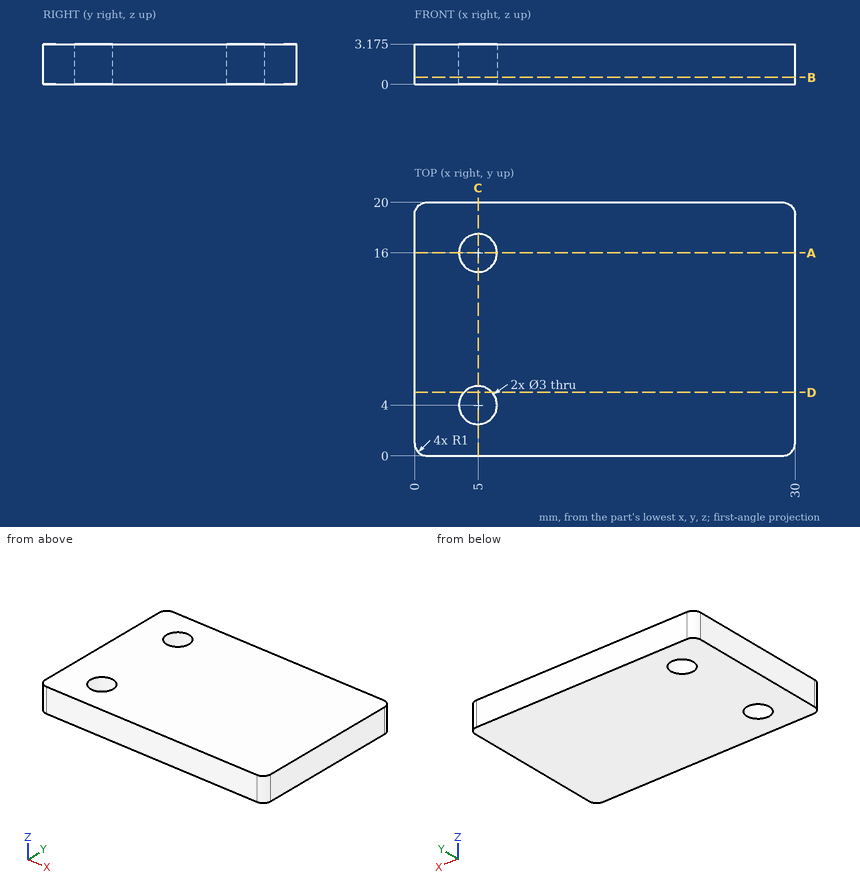
Study the drawing (mm; zero at the part's minimum x, y, z) and answer. Give positions to 0.01 mm unless a question says otherwise; leave off trailing zeros. Write each loop counter-clockwise with the first axis right and the second up, starting at its lowest first coordinate (ties: lowest second). Pieces come first, ordered by that corner, then holes. Notation, with made-up numbers: (-13, -1.5) - (7, -1.5) arc R24 ccw to (7, 10.5) - close; hole circle Ø11 at (69, 34.5). An arc over 180 degrees is marked (long way). One line per question, with ' | ' between items. Start each with the question number.
1. Section D-D, the plane y = 5 is taken. Determine the outline of the cut face in (x, z) (3 decimals), then the cut area to 3 significant figures.
2. Section B-B, the plane z = 0.55 is taken. Determine the outline of the cut face in (x, y), then the cut area to 3 significant figures.
3. Straight lines are drawn through the part: line 1 (Y direction, x = 5, z = 1.7); line 2 (X direction, y = 2.75, z = 3.05); line 3 (X direction, y = 16.75, z = 1.6). For each, find the intervals that lie inside material, in ascending order.
4. Section C-C, the plane x = 5 is taken. Determine the outline of the cut face in (y, z) (3 decimals).
5. Section A-A, the plane y = 16 is taken. Determine the outline of the cut face in (x, z) (3 decimals), then the cut area to 3 significant figures.
Result:
1) outline: (0, 0) - (3.882, 0) - (3.882, 3.175) - (0, 3.175) - close; (6.118, 0) - (30, 0) - (30, 3.175) - (6.118, 3.175) - close | area: 88.2 mm2
2) outline: (0, 1) arc R1 ccw to (1, 0) - (29, 0) arc R1 ccw to (30, 1) - (30, 19) arc R1 ccw to (29, 20) - (1, 20) arc R1 ccw to (0, 19) - close; hole circle Ø3 at (5, 4); hole circle Ø3 at (5, 16) | area: 585 mm2
3) line 1: y = 0 to 2.5, 5.5 to 14.5, 17.5 to 20 | line 2: x = 0 to 4.17, 5.83 to 30 | line 3: x = 0 to 3.7, 6.3 to 30
4) outline: (0, 0) - (2.5, 0) - (2.5, 3.175) - (0, 3.175) - close; (5.5, 0) - (14.5, 0) - (14.5, 3.175) - (5.5, 3.175) - close; (17.5, 0) - (20, 0) - (20, 3.175) - (17.5, 3.175) - close
5) outline: (0, 0) - (3.5, 0) - (3.5, 3.175) - (0, 3.175) - close; (6.5, 0) - (30, 0) - (30, 3.175) - (6.5, 3.175) - close | area: 85.7 mm2
